from build123d import *

# Parameters (mm, degrees)
F_3_8_CLEARANCE_HOLE1_D = 10.0838
CIRPATTERN1_COUNT       = 10


with BuildPart() as part:
    # Sketch1 → Revolve1 (revolve)
    with BuildSketch(Plane.XY, mode=Mode.PRIVATE) as revolve1_sk:
        Polygon((0, 76.2), (6.35, 76.2), (6.35, 57.15), (267.208, 57.15), (267.208, 53.34), (0, 53.34), align=None)
    revolve(revolve1_sk.sketch.rotate(Axis((0, 0, 0), (1, 0, 0)), 90), axis=Axis((0, 0, 0), (1, 0, 0)))

    # 3/8 Clearance Hole1 (through all)
    with Locations(Plane(origin=(6.35, 0, -67.31), x_dir=(0, 0, 1), z_dir=(1, 0, 0))):
        with Locations((0, 0)):
            f_3_8_clearance_hole1 = Hole(F_3_8_CLEARANCE_HOLE1_D / 2)

    # CirPattern1: 3/8 Clearance Hole1 ×10 about axis
    cirpattern1_axis = Axis((0, 0, 0), (1, 0, 0))
    for i in range(1, CIRPATTERN1_COUNT):
        add(f_3_8_clearance_hole1.rotate(cirpattern1_axis, i * 360 / CIRPATTERN1_COUNT), mode=Mode.SUBTRACT)


solid = part.part
Verification items for the finished model (mm, model axes). A direction names the side the tool comes from. Round coordinates to 2 decimals unless told otherwise and drop trailing zeros. Loops run counter-clockwise (first coordinate to the right, second up) from the corner with the lowest first, then second, coordinate; pieces in that order, holes last. Notation, with made-up numbers: (-12, 22) - (6, 22) arc R17 ccw to (6, 39) - close; hole circle Ø3 at (-29, 15). An arc over 180 degrees is marked (long way). Use a Markdown table: item, result. Add a question column.
1. Section check B-B, the plane z = 39.5. Record the boundary of the cut face in (x, y), plus the area to 3 significant figures.
2. Section check D-D, the plane x = 214. Record the boundary of the cut face in (y, z), plus the area to 3 significant figures.
3. Section check A-A, the plane y = 0. Record the boundary of the cut face in (x, z), plus the area to 3 significant figures.
4. Section check C-C, the plane y = -20.5. Record the boundary of the cut face in (x, z).
5. Gauge pin test, flat ends, axial feed: pin 1 (8 mm diameter, centred on x = 138.5, z = 48, fed in from +Y); pin 2 (1 mm diameter, centred on x = 87, y = -9.5, fed in from -Z); pin 3 (1 mm diameter, centred on x = 166.5, y = -42.5, fed in from +Z); pin 4 (6 mm diameter, centred on y = 0, z = 67.31, fed in from +X). Record the tip position at first contact, or that the pin passes through.
6. Thickness scan on probe 1 along Y at (x, z) = (29.5, 42); probe 2 along X at (y, z) = (48.5, 37.5); probe 3 along Z at (x, y) = (92, -21.5). Record the ranges inside material, lowest first. Write a range as [from, to].
7. Access from +Z, -Z, +X, -X, +Y, -Y to the whole of each face (thin tool, end or side, straight path). Record for faces 4 (the face through (3.13, -1.51, -72.12)), 5 (the face through (6.35, -57, 11)).
8. Release check for a two-part mould opening along Y. For faces 1 (the face through (0, -29, 46)), 2 (the face through (131.734, -52.886, -6.944)), 3 (the face through (138.605, -2.513, -57.095)) record: released by +Y, released by -Y, zero draft, split by the parting line, or undercut.
Checks:
| question | item | result |
|---|---|---|
| 1 | outline | (0, -65.16) - (6.35, -65.16) - (6.35, -41.3) - (267.21, -41.3) - (267.21, -35.85) - (0, -35.85) - close; (0, 35.85) - (267.21, 35.85) - (267.21, 41.3) - (6.35, 41.3) - (6.35, 65.16) - (0, 65.16) - close |
| 1 | area | 3,220 mm^2 |
| 2 | outline | circle Ø114.3 at (0, 0); hole circle Ø106.68 at (0, 0) |
| 2 | area | 1,320 mm^2 |
| 3 | outline | (0, -76.2) - (6.35, -76.2) - (6.35, -72.35) - (0, -72.35) - close; (0, -62.27) - (6.35, -62.27) - (6.35, -57.15) - (267.21, -57.15) - (267.21, -53.34) - (0, -53.34) - close; (0, 53.34) - (267.21, 53.34) - (267.21, 57.15) - (6.35, 57.15) - (6.35, 62.27) - (0, 62.27) - close; (0, 72.35) - (6.35, 72.35) - (6.35, 76.2) - (0, 76.2) - close |
| 3 | area | 2,150 mm^2 |
| 4 | outline | (0, -73.39) - (6.35, -73.39) - (6.35, -53.35) - (267.21, -53.35) - (267.21, -49.24) - (0, -49.24) - close; (0, 49.24) - (267.21, 49.24) - (267.21, 53.35) - (6.35, 53.35) - (6.35, 73.39) - (0, 73.39) - close |
| 5 | pin 1 | stops at y = 36.47 |
| 5 | pin 2 | stops at z = -56.44 |
| 5 | pin 3 | stops at z = 38.76 |
| 5 | pin 4 | passes through |
| 6 | probe 1 | y = [-38.76, -32.88], [32.88, 38.76] |
| 6 | probe 2 | x = [0, 6.35] |
| 6 | probe 3 | z = [-52.95, -48.82], [48.82, 52.95] |
| 7 | face 4 | +X, -X |
| 7 | face 5 | +X |
| 8 | face 1 | zero draft |
| 8 | face 2 | undercut |
| 8 | face 3 | split by the parting line |
